```python
from build123d import *

# Parameters (mm, degrees)
CROQUIS2_R              = 18.75
SALIENTE_EXTRUIR1_DEPTH = 129.5
CORTAR_EXTRUIR1_START   = -28.5
CROQUIS3_R              = 18.75
CROQUIS3_R_2            = 4
CORTAR_EXTRUIR1_DEPTH   = 28.5
CROQUIS4_W              = 66
CROQUIS4_H              = 42
SALIENTE_EXTRUIR2_DEPTH = 29
CROQUIS5_R              = 2.4
CORTAR_EXTRUIR2_DEPTH   = 109.309741021
CROQUIS6_R              = 2.25
CORTAR_EXTRUIR3_DEPTH   = 141.083011104
CORTAR_EXTRUIR4_DEPTH   = 12
REDONDEO1_R             = 10
CORTAR_EXTRUIR5_START   = -22
CORTAR_EXTRUIR5_DEPTH   = 22
SALIENTE_EXTRUIR3_START = -3
CROQUIS9_R              = 2.4
SALIENTE_EXTRUIR3_DEPTH = 3
CORTAR_EXTRUIR6_DEPTH   = 3


with BuildPart() as part:
    # Croquis2 → Saliente-Extruir1 (new body)
    with BuildSketch(Plane.XY):
        Circle(CROQUIS2_R)
    extrude(amount=SALIENTE_EXTRUIR1_DEPTH)

    # Croquis3 → Cortar-Extruir1 (cut)
    with BuildSketch(Plane.XY.offset(129.5).offset(CORTAR_EXTRUIR1_START)):
        Circle(CROQUIS3_R)
        Circle(CROQUIS3_R_2, mode=Mode.SUBTRACT)
    extrude(amount=CORTAR_EXTRUIR1_DEPTH, mode=Mode.SUBTRACT)

    # Croquis4 → Saliente-Extruir2 (add)
    with BuildSketch(Plane.XY.offset(101)):
        Rectangle(CROQUIS4_W, CROQUIS4_H)
    extrude(amount=-SALIENTE_EXTRUIR2_DEPTH)

    # Croquis5 → Cortar-Extruir2 (cut, through all)
    with BuildSketch(Plane.XY.offset(101)):
        with Locations((-26, 6)):
            Circle(CROQUIS5_R)
        with Locations((-26, -6)):
            Circle(CROQUIS5_R)
        with Locations(Location((26, -6, 0), (0, 0, 180))):
            Circle(CROQUIS5_R)
        with Locations(Location((26, 6, 0), (0, 0, 180))):
            Circle(CROQUIS5_R)
        with BuildLine():
            Line((-33, 6), (-33, 21))
            Line((-33, 21), (-20.899494937, 21))
            Line((-20.899494937, 21), (-30.949747468, 10.949747468))
            ThreePointArc((-30.949747468, 10.949747468), (-32.467156728, 8.678784027), (-33, 6))
        make_face()
        with BuildLine():
            Line((33, 21), (20.899494937, 21))
            Line((20.899494937, 21), (30.949747468, 10.949747468))
            ThreePointArc((30.949747468, 10.949747468), (32.467156728, 8.678784027), (33, 6))
            Line((33, 6), (33, 21))
        make_face()
    extrude(amount=-CORTAR_EXTRUIR2_DEPTH, mode=Mode.SUBTRACT)

    # Croquis6 → Cortar-Extruir3 (cut, through all)
    with BuildSketch(Plane.XZ.offset(21)):
        with Locations((-26, 92)):
            Circle(CROQUIS6_R)
        with Locations((-26, 80)):
            Circle(CROQUIS6_R)
        with Locations((26, 80)):
            Circle(CROQUIS6_R)
        with Locations((26, 92)):
            Circle(CROQUIS6_R)
    extrude(amount=-CORTAR_EXTRUIR3_DEPTH, mode=Mode.SUBTRACT)

    # Croquis7 → Cortar-Extruir4 (cut)
    with BuildSketch(Plane(origin=(33, 0, 0), x_dir=(0, 0, -1), z_dir=(1, 0, 0))):
        Polygon((-97, 21), (-97, -13), (-75, -13), (-75, -1.5), (-72, -1.5), (-72, 21), align=None)
    cortar_extruir4 = extrude(amount=-CORTAR_EXTRUIR4_DEPTH, mode=Mode.SUBTRACT)

    # Simetría1: Cortar-Extruir4 across plane
    add(cortar_extruir4.mirror(Plane(origin=(0, 0, 0), x_dir=(0, 0, 1), z_dir=(1, 0, 0))), mode=Mode.SUBTRACT)

    # Redondeo1
    redondeo1_edges = [part.edges().sort_by_distance(p)[0] for p in [
        (-20.899494937, 21, 86.5),
        (20.899494937, 21, 86.5),
    ]]
    fillet(redondeo1_edges, radius=REDONDEO1_R)

    # Croquis8 → Cortar-Extruir5 (cut)
    with BuildSketch(Plane.XY.offset(129.5).offset(CORTAR_EXTRUIR5_START)):
        with BuildLine():
            Line((-2.439487651, 3.17), (2.439487651, 3.17))
            ThreePointArc((2.439487651, 3.17), (0, 4), (-2.439487651, 3.17))
        make_face()
    extrude(amount=CORTAR_EXTRUIR5_DEPTH, mode=Mode.SUBTRACT)

    # Croquis9 → Saliente-Extruir3 (add)
    with BuildSketch(Plane(origin=(0, 0, 72), x_dir=(-1, 0, 0), z_dir=(0, 0, -1)).offset(SALIENTE_EXTRUIR3_START)):
        with Locations(Location((26, -6, 0), (0, 0, 180))):
            Circle(CROQUIS9_R)
        with Locations(Location((-26, -6, 0), (0, 0, 180))):
            Circle(CROQUIS9_R)
    extrude(amount=SALIENTE_EXTRUIR3_DEPTH)

    # Croquis10 → Cortar-Extruir6 (cut)
    with BuildSketch(Plane(origin=(0, 0, 72), x_dir=(-1, 0, 0), z_dir=(0, 0, -1))):
        Polygon((-21, -1.5), (-33, -13.5), (-33, -1.5), align=None)
        Polygon((33, -1.5), (21, -1.5), (33, -13.5), align=None)
    extrude(amount=-CORTAR_EXTRUIR6_DEPTH, mode=Mode.SUBTRACT)


solid = part.part
```
Geometry check sheet. Reference: the model listing, model coordinates, mm. A direction names the side the tool comes from. Coordinates: 2 decimals unless noted, no trailing zeros. Order: outer loops, then holes, each group sorted by start corner. A loop starts at its lowest first (then second) coordinate and runs counter-clockwise, first axis right, second up.
Item 1: Tool access check on faces 4 (the flat face through (-21, 4, 85)), 5 (the flat face through (26.9, -7.4, 73.5)), 6 (the cylindrical face through (-0.867, -3.905, 115.05)), 7 (the cylindrical face through (28.398, 5.894, 99.028)), 8 (the flat face through (27, 0, 97)). Record the directions out of +Z, -Z, +X, -X, +Y, -Y that give a thin tool (end or side, any length) a straight path to the whole face; none if there is none.
Item 2: Mould release check, pull along Z, two halves, no side actions. Record for faces 1 (the flat face through (0, -20, 72)), 2 (the cylindrical face through (25.512, -17.056, 77.804)), 3 (the cylindrical face through (18.868, 20.775, 86.297)): released by +Z, released by -Z, zero draft, split by the parting line, or undercut.
Item 3: Section check D-D (x = -26). Enter the section's corners in (y, z).
Item 4: Section check B-B (x = 0). Enter the section's corners in (y, z), plus the area to 3 significant figures.
Item 5: Section check C-C (y = -15). Enter the section's corners in (x, z).
Item 6: Section check A-A (z = 85). Enter the section's corners in (x, y), plus the area to 3 significant figures.
Item 7: Scan lines: line 1 along Z through (x, y) = (26, -18.5); line 2 along Z through (x, y) = (-26.5, -1.5); line 3 along Z through (x, y) = (-11, 3.5). Record each from-to range of solid material in increasing order.
Item 8: Depth check by flat-ended pin: pin 1 (9 mm diameter, centred on x = 28.5, y = -8.5, fed in from +Z); pin 2 (3 mm diameter, centred on x = 20, z = 71.5, fed in from +Y); pin 3 (6 mm diameter, centred on x = 26, z = 80, fed in from +Y). Enter the tip coordinate at first touch or a pass-through.
Check sheet entries:
1. face 4: -X, +Y
1. face 5: -Z, +X, +Y
1. face 6: +Z
1. face 7: +Z, -Z
1. face 8: +X, +Y
2. face 1: released by -Z
2. face 2: undercut
2. face 3: zero draft
3. outline: (-21, 72) - (-6.5, 72) - (-6.5, 75) - (-13, 75) - (-13, 77.75) - (-21, 77.75) - close; (-21, 82.25) - (-13, 82.25) - (-13, 89.75) - (-21, 89.75) - close; (-21, 94.25) - (-13, 94.25) - (-13, 97) - (-8.4, 97) - (-8.4, 101) - (-21, 101) - close; (-3.6, 97) - (3.6, 97) - (3.6, 101) - (-3.6, 101) - close; (8.4, 97) - (15.9, 97) - (15.9, 101) - (8.4, 101) - close
4. outline: (-21, 72) - (-18.75, 72) - (-18.75, 0) - (18.75, 0) - (18.75, 72) - (21, 72) - (21, 101) - (4, 101) - (4, 107.5) - (3.17, 107.5) - (3.17, 129.5) - (-4, 129.5) - (-4, 101) - (-21, 101) - close
4. area: 4,130 mm2
5. outline: (-33, 72) - (-11.25, 72) - (-11.25, 0) - (11.25, 0) - (11.25, 72) - (33, 72) - (33, 101) - (-33, 101) - close; hole circle Ø4.5 at (-26, 80); hole circle Ø4.5 at (-26, 92); hole circle Ø4.5 at (26, 80); hole circle Ø4.5 at (26, 92)
6. outline: (-33, -21) - (33, -21) - (33, -13) - (21, -13) - (21, 20.06) arc R10 ccw to (16.76, 21) - (-16.76, 21) arc R10 ccw to (-21, 20.06) - (-21, -13) - (-33, -13) - close
6. area: 1,950 mm2
7. line 1: z = 72 to 77.75, 82.25 to 89.75, 94.25 to 101
7. line 2: z = 97 to 101
7. line 3: z = 0 to 101
8. pin 1: stops at z = 101
8. pin 2: stops at y = 20.83
8. pin 3: stops at y = -13
